Model file for the job. Use its own axes, mm. A direction names the side the tool comes from. Round coordinates to 2 decimals unless told otherwise and drop trailing zeros. Loops run counter-clockwise (first coordinate to the right, second up) from the corner with the lowest first, then second, coordinate; pieces in that order, holes last. Notation, with made-up numbers: (-2, -37) -> (13, -37) arc R25 ccw to (13, -20) -> close; hole circle Ø2 at (1, 38.25). An arc over 180 degrees is marked (long way). Use a Markdown table: item, result.
from build123d import *

# Parameters (mm, degrees)
SKETCH_1_R          = 5
SKETCH_1_R_2        = 2.5
EXTRUDE_1_DEPTH     = 4.3
SKETCH_3_R          = 1.825
CUT_EXTRUDE_1_DEPTH = 1.8
CUT_EXTRUDE_2_REACH = 36.091
SKETCH_4_R          = 0.1


with BuildPart() as part:
    # 스케치1 → 보스-돌출1 (new body)
    # profile 1 of 2: a face of its own
    with BuildSketch(Plane.XY):
        with BuildLine():
            ThreePointArc((5, 0), (0, -5), (-5, 0))
            Line((-5, 0), (-5, -2.326474397))
            Line((-5, -2.326474397), (0.754164722, -7.377840375))
            Line((0.754164722, -7.377840375), (0.754164722, -29.519890116))
            Line((0.754164722, -29.519890116), (2.889052882, -29.519890116))
            Line((2.889052882, -29.519890116), (3.452626944, -25.890848407))
            Line((3.452626944, -25.890848407), (7.880357437, -17.740939791))
            Line((7.880357437, -17.740939791), (7.880357437, -12.211059606))
            Line((7.880357437, -12.211059606), (6.40208237, -11.079255258))
            Line((6.40208237, -11.079255258), (6.40208237, -3.237610212))
            ThreePointArc((6.40208237, -3.237610212), (6.694975589, -2.530503431), (7.40208237, -2.237610212))
            Line((7.40208237, -2.237610212), (18.063612226, -2.237610212))
            Line((18.063612226, -2.237610212), (19.056002599, 4.757997197))
            Line((19.056002599, 4.757997197), (1.536705134, 4.757997197))
            ThreePointArc((1.536705134, 4.757997197), (4.04249463, 2.942488261), (5, 0))
        make_face()
    # profile 2 of 2: a face of its own
    with BuildSketch(Plane.XY):
        Circle(SKETCH_1_R)
        with Locations(Location((0, 0, 0), (0, 0, 180))):
            Circle(SKETCH_1_R_2, mode=Mode.SUBTRACT)
    extrude(amount=EXTRUDE_1_DEPTH)

    # 스케치3 → 컷-돌출1 (cut)
    with BuildSketch(Plane.ZY.offset(-0.754164722)):
        with Locations((2.174780249, -27.020012931)):
            Circle(SKETCH_3_R)
    extrude(amount=-CUT_EXTRUDE_1_DEPTH, mode=Mode.SUBTRACT)

    # 컷-돌출2: up to this plane
    cut_extrude_2_end = Plane(origin=(7.297372122, -1.133249487, 4.3), z_dir=(-0.9881554576984991, 0.15345615471746255, 0))
    # 스케치4 → 컷-돌출2 (cut, up to the surface)
    with BuildSketch(Plane.ZY.offset(-2.554164722), mode=Mode.PRIVATE) as cut_extrude_2_sk1:
        with Locations((2.174780249, -28.345012931)):
            Circle(SKETCH_4_R)
    cut_extrude_2_tool1 = split(extrude(cut_extrude_2_sk1.sketch, amount=-CUT_EXTRUDE_2_REACH, mode=Mode.PRIVATE), bisect_by=cut_extrude_2_end, keep=Keep.BOTH, mode=Mode.PRIVATE)
    add(cut_extrude_2_tool1.solids().sort_by_distance((2.554165, -28.345013, 2.17478))[0], mode=Mode.SUBTRACT)


solid = part.part
Q1. Tool access for faces 1 (the face through (-3, 4, 2)), 2 (the face through (2.5, -0.1, 2.1)), 3 (the face through (0.754, -16, 2)), 4 (the face through (6.402, -7, 2)), 5 (the face through (7.88, -15, 2)): list every direction of +Z, -Z, +X, -X, +Y, -Y with a clear straight run to the whole face (end or side of a thin tool).
Results list:
| item | result |
|---|---|
| face 1 | +Z, -Z, +Y |
| face 2 | +Z, -Z |
| face 3 | +Z, -Z, -X, -Y |
| face 4 | +Z, -Z, +X |
| face 5 | +Z, -Z, +X, -Y |
Q2. Drill centre lines: L1, parallel to Y at x = 11.5, z = 2.8; L2, parallel to X at y = -12.5, z = 0.7; L3, parallel to Y at x = 7, z = 2.95. Where is each one in solid material? Low to high. Write a range as from..to.
Results list:
| item | result |
|---|---|
| L1 | y = -2.24..4.76 |
| L2 | x = 0.75..7.88 |
| L3 | y = -19.36..-11.54, -2.32..4.76 |
Q3. Flat gauge pins, fed straight in: pin 1 (2 mm diameter, centred on y = -9, z = 1.5, fed in from +X); pin 2 (1.3 mm diameter, centred on x = 14, z = 1.5, fed in from +Y); pin 3 (2 mm diameter, centred on y = -8.5, z = 1.5, fed in from -X). Where does each tip first touch, or does it go through?
Results list:
| item | result |
|---|---|
| pin 1 | stops at x = 6.4 |
| pin 2 | stops at y = 4.76 |
| pin 3 | stops at x = 0.75 |
Q4. Band-saw the part on A-A, the plane x = 0. Give the cut face in (y, z).
Results list:
| item | result |
|---|---|
| outline | (-6.72, 0) -> (-2.5, 0) -> (-2.5, 4.3) -> (-6.72, 4.3) -> close; (2.5, 0) -> (5, 0) -> (5, 4.3) -> (2.5, 4.3) -> close |
Q5. Band-saw the part on B-B, the plane z = 1.2. Give the cut face in (x, y), plus the area to 3 significant figures.
Results list:
| item | result |
|---|---|
| outline | (-5, -2.33) -> (0.75, -7.38) -> (0.75, -25.48) -> (2.55, -25.48) -> (2.55, -28.56) -> (0.75, -28.56) -> (0.75, -29.52) -> (2.89, -29.52) -> (3.45, -25.89) -> (7.88, -17.74) -> (7.88, -12.21) -> (6.4, -11.08) -> (6.4, -3.24) arc R1 cw to (7.4, -2.24) -> (18.06, -2.24) -> (19.06, 4.76) -> (1.54, 4.76) arc R5 ccw to (-5, 0) -> close; hole circle Ø5 at (0, 0) |
| area | 296 mm² |
Q6. Band-saw the part on C-C, the plane y = -9.5. Give the cut face in (x, z).
Results list:
| item | result |
|---|---|
| outline | (0.75, 0) -> (6.4, 0) -> (6.4, 4.3) -> (0.75, 4.3) -> close |
Q7. Pull direction Z, two halves, no side cores. Call faces 6 (the face through (10, 4.758, 2)), 7 (the face through (4, -8, 4.3)), 8 (the face through (1.642, -25.481, 3.156)): released by +Z, released by -Z, zero draft, split by the parting line, or undercut.
Results list:
| item | result |
|---|---|
| face 6 | zero draft |
| face 7 | released by +Z |
| face 8 | undercut |
Q8. Band-saw the part on D-D, the plane x = 16.75. Give the cut face in (y, z).
Results list:
| item | result |
|---|---|
| outline | (-2.24, 0) -> (4.76, 0) -> (4.76, 4.3) -> (-2.24, 4.3) -> close |
